from build123d import *

# Parameters (mm, degrees)
CROQUIS1_R              = 105
SALIENTE_EXTRUIR1_DEPTH = 3
CORTAR_EXTRUIR1_START   = -3
CORTAR_EXTRUIR1_DEPTH   = 3
REDONDEO1_R             = 10
CROQUIS3_W              = 38
CROQUIS3_H              = 30
CORTAR_EXTRUIR2_DEPTH   = 149.522725677
MATRIZC2_COUNT          = 3
CORTAR_EXTRUIR3_DEPTH   = 148.302410171
CROQUIS5_R              = 1.5
CORTAR_EXTRUIR4_DEPTH   = 148.302410171
CROQUIS6_R              = 1.5
CORTAR_EXTRUIR5_DEPTH   = 148.302410171
CROQUIS7_R              = 1.5
CORTAR_EXTRUIR6_DEPTH   = 148.302410171
CROQUIS8_R              = 1.5
CORTAR_EXTRUIR8_DEPTH   = 10
CORTAR_EXTRUIR9_DEPTH   = 148.302410171
CROQUIS11_R             = 1.5
CORTAR_EXTRUIR10_DEPTH  = 148.302410171
CROQUIS12_R             = 1.5
CORTAR_EXTRUIR11_DEPTH  = 148.302410171
CROQUIS14_R             = 1.5
CORTAR_EXTRUIR15_DEPTH  = 148.302410171
CORTAR_EXTRUIR18_DEPTH  = 148.302410171
CROQUIS17_R             = 10
CORTAR_EXTRUIR19_DEPTH  = 148.302410171
CROQUIS19_R             = 1.5
CORTAR_EXTRUIR20_DEPTH  = 148.302410171
CROQUIS20_W             = 23
CROQUIS20_H             = 20
CORTAR_EXTRUIR21_DEPTH  = 148.302410171
CROQUIS21_R             = 1.5
CORTAR_EXTRUIR23_DEPTH  = 10
CROQUIS22_R             = 2
CORTAR_EXTRUIR24_DEPTH  = 148.302410171
CORTAR_EXTRUIR25_DEPTH  = 148.302410171
CROQUIS24_W             = 34
CROQUIS24_H             = 17
CORTAR_EXTRUIR26_DEPTH  = 148.302410171


with BuildPart() as part:
    # Croquis1 → Saliente-Extruir1 (new body)
    with BuildSketch(Plane(origin=(0, 0, 0), x_dir=(1, 0, 0), z_dir=(0, 1, 0))):
        with Locations(Location((0, 0, 0), (0, 0, 270))):
            Circle(CROQUIS1_R)
    extrude(amount=SALIENTE_EXTRUIR1_DEPTH)

    # Croquis2 → Cortar-Extruir1 (cut)
    with BuildSketch(Plane(origin=(0, 3, 0), x_dir=(1, 0, 0), z_dir=(0, 1, 0)).offset(CORTAR_EXTRUIR1_START)):
        with BuildLine():
            ThreePointArc((35.71668902, 98.738635424), (0, 68.738635424), (-35.71668902, 98.738635424))
            ThreePointArc((-35.71668902, 98.738635424), (0, 105), (35.71668902, 98.738635424))
        make_face()
    extrude(amount=CORTAR_EXTRUIR1_DEPTH, mode=Mode.SUBTRACT)

    # Redondeo1
    redondeo1_edges = [part.edges().sort_by_distance(p)[0] for p in [
        (-35.71668902, 1.5, -98.738635424),
        (35.71668902, 1.5, -98.738635424),
    ]]
    fillet(redondeo1_edges, radius=REDONDEO1_R)

    # Croquis3 → Cortar-Extruir2 (cut, through all)
    with BuildSketch(Plane(origin=(0, 3, 0), x_dir=(1, 0, 0), z_dir=(0, 1, 0))):
        with Locations((0, -90)):
            Rectangle(CROQUIS3_W, CROQUIS3_H)
    cortar_extruir2 = extrude(amount=-CORTAR_EXTRUIR2_DEPTH, mode=Mode.SUBTRACT)

    # MatrizC2: Cortar-Extruir2 ×3 about axis
    matrizc2_axis = Axis((0, 0, 0), (0, 1, 0))
    for i in range(1, MATRIZC2_COUNT):
        add(cortar_extruir2.rotate(matrizc2_axis, i * 360 / MATRIZC2_COUNT), mode=Mode.SUBTRACT)

    # Croquis4 → Cortar-Extruir3 (cut, through all)
    with BuildSketch(Plane(origin=(0, 3, 0), x_dir=(1, 0, 0), z_dir=(0, 1, 0))):
        Polygon((-88, -3), (-38, -3), (-38, -8), (-33, -8), (-33, -15), (-38, -15), (-38, -20), (-88, -20), (-88, -15), (-93, -15), (-93, -8), (-88, -8), align=None)
        Polygon((33, -15), (38, -15), (38, -20), (88, -20), (88, -15), (93, -15), (93, -8), (88, -8), (88, -3), (38, -3), (38, -8), (33, -8), align=None)
    extrude(amount=-CORTAR_EXTRUIR3_DEPTH, mode=Mode.SUBTRACT)

    # Croquis5 → Cortar-Extruir4 (cut, through all)
    with BuildSketch(Plane(origin=(0, 3, 0), x_dir=(1, 0, 0), z_dir=(0, 1, 0))):
        with Locations(Location((-90.5, -5.5, 0), (0, 0, 270))):
            Circle(CROQUIS5_R)
        with Locations(Location((90.5, -5.5, 0), (0, 0, 90))):
            Circle(CROQUIS5_R)
    extrude(amount=-CORTAR_EXTRUIR4_DEPTH, mode=Mode.SUBTRACT)

    # Croquis6 → Cortar-Extruir5 (cut, through all)
    with BuildSketch(Plane(origin=(0, 3, 0), x_dir=(1, 0, 0), z_dir=(0, 1, 0))):
        with Locations(Location((-90.5, -17.5, 0), (0, 0, 270))):
            Circle(CROQUIS6_R)
        with Locations(Location((90.5, -17.5, 0), (0, 0, 90))):
            Circle(CROQUIS6_R)
    extrude(amount=-CORTAR_EXTRUIR5_DEPTH, mode=Mode.SUBTRACT)

    # Croquis7 → Cortar-Extruir6 (cut, through all)
    with BuildSketch(Plane(origin=(0, 3, 0), x_dir=(1, 0, 0), z_dir=(0, 1, 0))):
        with Locations(Location((-35.5, -17.5, 0), (0, 0, 270))):
            Circle(CROQUIS7_R)
        with Locations(Location((35.5, -17.5, 0), (0, 0, 90))):
            Circle(CROQUIS7_R)
    extrude(amount=-CORTAR_EXTRUIR6_DEPTH, mode=Mode.SUBTRACT)

    # Croquis8 → Cortar-Extruir8 (cut)
    with BuildSketch(Plane(origin=(0, 3, 0), x_dir=(1, 0, 0), z_dir=(0, 1, 0))):
        with Locations(Location((-35.5, -5.5, 0), (0, 0, 270))):
            Circle(CROQUIS8_R)
        with Locations(Location((35.5, -5.5, 0), (0, 0, 270))):
            Circle(CROQUIS8_R)
    extrude(amount=-CORTAR_EXTRUIR8_DEPTH, mode=Mode.SUBTRACT)

    # Croquis10 → Cortar-Extruir9 (cut, through all)
    with BuildSketch(Plane(origin=(0, 3, 0), x_dir=(1, 0, 0), z_dir=(0, 1, 0))):
        Polygon((-3.5, 64), (3.5, 64), (3.5, 59), (8.5, 59), (8.5, 9), (3.5, 9), (3.5, 4), (-3.5, 4), (-3.5, 9), (-8.5, 9), (-8.5, 59), (-3.5, 59), align=None)
    extrude(amount=-CORTAR_EXTRUIR9_DEPTH, mode=Mode.SUBTRACT)

    # Croquis11 → Cortar-Extruir10 (cut, through all)
    with BuildSketch(Plane(origin=(0, 3, 0), x_dir=(1, 0, 0), z_dir=(0, 1, 0))):
        with Locations(Location((-6, 61.5, 0), (0, 0, 270))):
            Circle(CROQUIS11_R)
        with Locations(Location((6, 61.5, 0), (0, 0, 270))):
            Circle(CROQUIS11_R)
    extrude(amount=-CORTAR_EXTRUIR10_DEPTH, mode=Mode.SUBTRACT)

    # Croquis12 → Cortar-Extruir11 (cut, through all)
    with BuildSketch(Plane(origin=(0, 3, 0), x_dir=(1, 0, 0), z_dir=(0, 1, 0))):
        with Locations(Location((-6, 6.5, 0), (0, 0, 270))):
            Circle(CROQUIS12_R)
        with Locations(Location((6, 6.5, 0), (0, 0, 270))):
            Circle(CROQUIS12_R)
    extrude(amount=-CORTAR_EXTRUIR11_DEPTH, mode=Mode.SUBTRACT)

    # Croquis14 → Cortar-Extruir15 (cut, through all)
    with BuildSketch(Plane(origin=(0, 3, 0), x_dir=(1, 0, 0), z_dir=(0, 1, 0))):
        with Locations(Location((-19, -47.266645147, 0), (0, 0, 270))):
            Circle(CROQUIS14_R)
        with Locations(Location((-19, -62.266645147, 0), (0, 0, 270))):
            Circle(CROQUIS14_R)
        with Locations(Location((18.5, -47.266645147, 0), (0, 0, 270))):
            Circle(CROQUIS14_R)
        with Locations(Location((18.5, -62.266645147, 0), (0, 0, 270))):
            Circle(CROQUIS14_R)
    extrude(amount=-CORTAR_EXTRUIR15_DEPTH, mode=Mode.SUBTRACT)

    # Croquis16 → Cortar-Extruir18 (cut, through all)
    with BuildSketch(Plane(origin=(0, 3, 0), x_dir=(1, 0, 0), z_dir=(0, 1, 0))):
        with BuildLine():
            Line((-85.199337741, -32), (-30.199337741, -32))
            Line((-30.199337741, -32), (-30.199337741, -87))
            ThreePointArc((-30.199337741, -87), (-69.090210706, -70.890872965), (-85.199337741, -32))
        make_face()
        with BuildLine():
            Line((30.199337741, -32), (30.199337741, -87))
            ThreePointArc((30.199337741, -87), (69.090210706, -70.890872965), (85.199337741, -32))
            Line((85.199337741, -32), (30.199337741, -32))
        make_face()
    extrude(amount=-CORTAR_EXTRUIR18_DEPTH, mode=Mode.SUBTRACT)

    # Croquis17 → Cortar-Extruir19 (cut, through all)
    with BuildSketch(Plane(origin=(0, 3, 0), x_dir=(1, 0, 0), z_dir=(0, 1, 0))):
        with Locations(Location((-48, 74, 0), (0, 0, 270))):
            Circle(CROQUIS17_R)
        with Locations(Location((48, 74, 0), (0, 0, 90))):
            Circle(CROQUIS17_R)
    extrude(amount=-CORTAR_EXTRUIR19_DEPTH, mode=Mode.SUBTRACT)

    # Croquis19 → Cortar-Extruir20 (cut, through all)
    with BuildSketch(Plane(origin=(0, 3, 0), x_dir=(1, 0, 0), z_dir=(0, 1, 0))):
        with Locations(Location((-15, -35, 0), (0, 0, 270))):
            Circle(CROQUIS19_R)
        with Locations(Location((15, -35, 0), (0, 0, 270))):
            Circle(CROQUIS19_R)
        with Locations(Location((23.5, -13.5, 0), (0, 0, 270))):
            Circle(CROQUIS19_R)
        with Locations(Location((23.5, -26.5, 0), (0, 0, 270))):
            Circle(CROQUIS19_R)
        with Locations(Location((-23.5, -26.5, 0), (0, 0, 270))):
            Circle(CROQUIS19_R)
        with Locations(Location((-23.5, -13.5, 0), (0, 0, 270))):
            Circle(CROQUIS19_R)
        with Locations(Location((-15, -5, 0), (0, 0, 270))):
            Circle(CROQUIS19_R)
        with Locations(Location((15, -5, 0), (0, 0, 270))):
            Circle(CROQUIS19_R)
    extrude(amount=-CORTAR_EXTRUIR20_DEPTH, mode=Mode.SUBTRACT)

    # Croquis20 → Cortar-Extruir21 (cut, through all)
    with BuildSketch(Plane(origin=(0, 3, 0), x_dir=(1, 0, 0), z_dir=(0, 1, 0))):
        with Locations((-0.5, -55.766645147)):
            Rectangle(CROQUIS20_W, CROQUIS20_H)
    extrude(amount=-CORTAR_EXTRUIR21_DEPTH, mode=Mode.SUBTRACT)

    # Croquis21 → Cortar-Extruir23 (cut)
    with BuildSketch(Plane(origin=(0, 3, 0), x_dir=(1, 0, 0), z_dir=(0, 1, 0))):
        with Locations(Location((-62.637803669, 33.508141571, 0), (0, 0, 270))):
            Circle(CROQUIS21_R)
        with Locations(Location((-55.987803669, 45.026279442, 0), (0, 0, 270))):
            Circle(CROQUIS21_R)
        with Locations(Location((-28.274990748, 29.026279442, 0), (0, 0, 270))):
            Circle(CROQUIS21_R)
        with Locations(Location((-34.924990748, 17.508141571, 0), (0, 0, 270))):
            Circle(CROQUIS21_R)
        with Locations(Location((28.274990748, 29.026279442, 0), (0, 0, 270))):
            Circle(CROQUIS21_R)
        with Locations(Location((34.924990748, 17.508141571, 0), (0, 0, 270))):
            Circle(CROQUIS21_R)
        with Locations(Location((62.637803669, 33.508141571, 0), (0, 0, 270))):
            Circle(CROQUIS21_R)
        with Locations(Location((55.987803669, 45.026279442, 0), (0, 0, 270))):
            Circle(CROQUIS21_R)
    extrude(amount=-CORTAR_EXTRUIR23_DEPTH, mode=Mode.SUBTRACT)

    # Croquis22 → Cortar-Extruir24 (cut, through all)
    with BuildSketch(Plane(origin=(0, 3, 0), x_dir=(1, 0, 0), z_dir=(0, 1, 0))):
        with Locations(Location((-100.968056074, -2.540010349, 0), (0, 0, 270))):
            Circle(CROQUIS22_R)
        with Locations(Location((-52.683741526, 86.170896356, 0), (0, 0, 270))):
            Circle(CROQUIS22_R)
        with Locations(Location((48.284314549, 88.710906706, 0), (0, 0, 270))):
            Circle(CROQUIS22_R)
        with Locations(Location((100.968056074, 2.540010349, 0), (0, 0, 270))):
            Circle(CROQUIS22_R)
        with Locations(Location((52.683741526, -86.170896356, 0), (0, 0, 270))):
            Circle(CROQUIS22_R)
        with Locations(Location((-48.284314549, -88.710906706, 0), (0, 0, 270))):
            Circle(CROQUIS22_R)
    extrude(amount=-CORTAR_EXTRUIR24_DEPTH, mode=Mode.SUBTRACT)

    # Croquis23 → Cortar-Extruir25 (cut, through all)
    with BuildSketch(Plane(origin=(0, 3, 0), x_dir=(1, 0, 0), z_dir=(0, 1, 0))):
        Polygon((-62.258330249, 23.165408814), (-27.758330249, 82.921161675), (-10.437822174, 72.921161675), (-44.937822174, 13.165408814), align=None)
        Polygon((27.758330249, 82.921161675), (10.437822174, 72.921161675), (44.937822174, 13.165408814), (62.258330249, 23.165408814), align=None)
    extrude(amount=-CORTAR_EXTRUIR25_DEPTH, mode=Mode.SUBTRACT)

    # Croquis24 → Cortar-Extruir26 (cut, through all)
    with BuildSketch(Plane(origin=(0, 3, 0), x_dir=(1, 0, 0), z_dir=(0, 1, 0))):
        with Locations((0, -20)):
            Rectangle(CROQUIS24_W, CROQUIS24_H)
    extrude(amount=-CORTAR_EXTRUIR26_DEPTH, mode=Mode.SUBTRACT)


solid = part.part
Work out the finished part from the listing and answer in its coordinate system (mm). A direction names the side the tool comes from. Round coordinates to 2 decimals unless told otherwise and drop trailing zeros.
1) A tool of negligible diameter and unlimited length cuts with its end or side. For faces 1 (the flat face through (67.86, 1.52, -61.12)), 2 (the cylindrical face through (-30.7, 1.5, -85.7)), 3 (the flat face through (-67.86, 1.52, -61.12)), 4 (the cylindrical face through (64.7, 1.5, -82.7)), 5 (the flat face through (-64.82, 1.52, -37.73)), from which of +Z, -Z, +X, -X, +Y, -Y can it reach the whole face along a straight path? Write none if from no direction.
2) A cutting plane is placed at A-A (y = 1.65). Give the number of separate pieces and of enclosed holes in the cut face, plus the area to 3 significant figures.
3) Straight lines are drawn through the part: line 1 (Z direction, x = 2, y = 1.65); line 2 (X direction, y = 2.95, z = -7); line 3 (X direction, y = 1, z = -52.5). For each, find the intervals that lie inside material, in ascending order.
4) Given pin 1 Ø1.5 at (y, z) = (1, -60.5) entering from -X; pin 2 Ø2.5 at (x, z) = (15, 35) entering from -Y; pin 3 Ø1.5 at (x, y) = (-68.5, 2) entering from +Z; pin 4 Ø1.5 at (y, z) = (2, 15.5) entering from -X, each flat-ended and moving along its own axis, determine where each tip first touches the part or whether it passes through.
5) The mould has two halves that part along Z. Classify faces 6 (the cylindrical face through (30.75, 1.48, -85.78)), 7 (the cylindrical face through (-68.66, 1.521, 71.316)), 8 (the flat face through (1, 3, 3)), 9 (the cylindrical face through (-91.562, 1.479, 51.395)): pulls with the +Z half, pulls with the -Z half, needs draft (parallel to the pull), parting line crosses it, or undercut.
Completed:
1. face 1: +X, +Y, -Y
1. face 2: -Z, +Y, -Y
1. face 3: -X, +Y, -Y
1. face 4: -Z, +X, +Y, -Y
1. face 5: +Y, -Y
2. separate pieces: 1
2. enclosed holes: 47
2. area: 17,200 mm2
3. line 1: z = -68.79 to -64, -4 to 11.5, 28.5 to 45.77, 65.77 to 75
3. line 2: x = -104.77 to -7.41, -4.59 to -3.5, 3.5 to 4.59, 7.41 to 104.77
3. line 3: x = -56.29 to -45.32, -22.23 to -8.5, 8.5 to 22.23, 45.32 to 56.29
4. pin 1: stops at x = -68.09
4. pin 2: passes through
4. pin 3: stops at z = 80.22
4. pin 4: stops at x = -103.96
5. face 6: pulls with the -Z half
5. face 7: undercut
5. face 8: needs draft
5. face 9: parting line crosses it
